```python
from build123d import *

# Parameters (mm, degrees)
SKETCH001_W   = 32
SKETCH001_H   = 42
SKETCH001_R   = 1.5
SKETCH001_W_2 = 12.3
SKETCH001_H_2 = 23.1
EXTRUDE_DEPTH = 1.5
FILLET_R      = 20


with BuildPart() as part:
    # Sketch001 → Extrude (new body)
    with BuildSketch(Plane.XY):
        with Locations((-0.15, 0)):
            Rectangle(SKETCH001_W, SKETCH001_H)
        with Locations((0, 14.1)):
            Circle(SKETCH001_R, mode=Mode.SUBTRACT)
        with Locations((0, -14.1)):
            Circle(SKETCH001_R, mode=Mode.SUBTRACT)
        Rectangle(SKETCH001_W_2, SKETCH001_H_2, mode=Mode.SUBTRACT)
        with BuildLine():
            ThreePointArc((-9.15, 14), (-11.15, 16), (-13.15, 14))
            Line((-13.15, 14), (-13.15, -14))
            ThreePointArc((-13.15, -14), (-11.15, -16), (-9.15, -14))
            Line((-9.15, 14), (-9.15, -14))
        make_face(mode=Mode.SUBTRACT)
    extrude(amount=EXTRUDE_DEPTH)

    # Fillet
    fillet_edges = [part.edges().sort_by_distance(p)[0] for p in [
        (15.85, 21, 0.75),
        (15.85, -21, 0.75),
    ]]
    fillet(fillet_edges, radius=FILLET_R)


solid = part.part
```
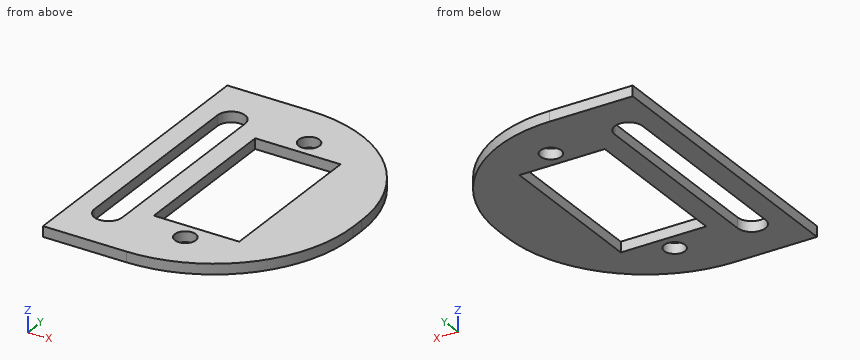
Read the model definition and answer for the solid it produces. Units are mm, in the model's axes. Give positions to 0.01 mm unless a question says otherwise; leave off trailing zeros. Loops run counter-clockwise (first coordinate to the right, second up) from the corner with the lowest first, then second, coordinate; pieces in that order, holes last.
Item 1: Find the intervals of material crossed by line 1 along X through (y, z) = (-1, 1.4); line 2 along Y through (x, z) = (-4.5, 1); line 3 along Y through (x, z) = (0.5, 0.2), in increasing order.
Item 2: This flat-tipped pin is pushed along its axis until it touches: pin 1 Ø1.8 at (x, y) = (0, 14.1) entering from -Z. Where does it stop, or does it pass through?
Item 3: The part is cut by section B-B (y = 12). Write down the section's boundary in (x, z).
Item 4: The part is cut by section C-C (z = 0.45). Write down the section's boundary in (x, y).
Item 5: The part is cut by section D-D (x = 0). Write down the section's boundary in (y, z), and give its area (3 significant figures).
Item 6: The part is cut by section A-A (x = -11.15). Write down the section's boundary in (y, z), and give its area (3 significant figures).
Taken from the geometry:
1. line 1: x = -16.15 to -13.15, -9.15 to -6.15, 6.15 to 15.85
1. line 2: y = -21 to -11.55, 11.55 to 21
1. line 3: y = -20.45 to -15.51, -12.69 to -11.55, 11.55 to 12.69, 15.51 to 20.45
2. pin 1: passes through
3. outline: (-16.15, 0) - (-13.15, 0) - (-13.15, 1.5) - (-16.15, 1.5) - close; (-9.15, 0) - (12.55, 0) - (12.55, 1.5) - (-9.15, 1.5) - close
4. outline: (-16.15, -21) - (-4.15, -21) arc R20 ccw to (15.85, -1) - (15.85, 1) arc R20 ccw to (-4.15, 21) - (-16.15, 21) - close; hole (-13.15, -14) arc R2 ccw to (-9.15, -14) - (-9.15, 14) arc R2 ccw to (-13.15, 14) - close; hole (-6.15, -11.55) - (6.15, -11.55) - (6.15, 11.55) - (-6.15, 11.55) - close; hole circle Ø3 at (0, -14.1); hole circle Ø3 at (0, 14.1)
5. outline: (-20.56, 0) - (-15.6, 0) - (-15.6, 1.5) - (-20.56, 1.5) - close; (-12.6, 0) - (-11.55, 0) - (-11.55, 1.5) - (-12.6, 1.5) - close; (11.55, 0) - (12.6, 0) - (12.6, 1.5) - (11.55, 1.5) - close; (15.6, 0) - (20.56, 0) - (20.56, 1.5) - (15.6, 1.5) - close
5. area: 18.0 mm2
6. outline: (-21, 0) - (-16, 0) - (-16, 1.5) - (-21, 1.5) - close; (16, 0) - (21, 0) - (21, 1.5) - (16, 1.5) - close
6. area: 15.0 mm2
